```python
from build123d import *

# Parameters (mm, degrees)
F0_R     = 0.8
F0_R_2   = 1.5
F0_R_3   = 1.25
F1_DEPTH = 2


with BuildPart() as f1:
    # F0 (on Top) → F1 (new body)
    with BuildSketch(Plane.XY):
        with BuildLine():
            Line((10.009608, -5.875233), (10.009608, 5.875233))
            ThreePointArc((10.009608, 5.875233), (10.10321, 6.479919), (10.375253, 7.028005))
            Line((10.375253, 7.028005), (11.773889, 8.782295))
            ThreePointArc((11.773889, 8.782295), (12.209984, 10.04744), (11.750731, 11.304364))
            Line((11.750731, 11.304364), (10.320118, 13.032675))
            ThreePointArc((10.320118, 13.032675), (10.044588, 13.582548), (9.949174, 14.190143))
            Line((9.949174, 14.190143), (8.682091, 25.56351))
            ThreePointArc((8.682091, 25.56351), (8.678182, 25.607343), (8.676205, 25.651306))
            ThreePointArc((8.676205, 25.651306), (6.95314, 27.312167), (5.276671, 25.604284))
            ThreePointArc((5.276671, 25.604284), (5.276621, 25.588507), (5.276322, 25.572732))
            Line((5.276322, 25.572732), (5.024577, 16.189424))
            ThreePointArc((5.024577, 16.189424), (4.40399, 14.772505), (2.970938, 14.190143))
            Line((2.970938, 14.190143), (-2.970938, 14.190143))
            ThreePointArc((-2.970938, 14.190143), (-4.40399, 14.772505), (-5.024577, 16.189424))
            Line((-5.024577, 16.189424), (-5.276322, 25.572732))
            ThreePointArc((-5.276322, 25.572732), (-5.276621, 25.588507), (-5.276671, 25.604284))
            ThreePointArc((-5.276671, 25.604284), (-6.95314, 27.312167), (-8.676205, 25.651306))
            ThreePointArc((-8.676205, 25.651306), (-8.678182, 25.607343), (-8.682091, 25.56351))
            Line((-8.682091, 25.56351), (-9.949174, 14.190143))
            ThreePointArc((-9.949174, 14.190143), (-10.044588, 13.582548), (-10.320118, 13.032675))
            Line((-10.320118, 13.032675), (-11.750731, 11.304364))
            ThreePointArc((-11.750731, 11.304364), (-12.209984, 10.04744), (-11.773889, 8.782295))
            Line((-11.773889, 8.782295), (-10.375253, 7.028005))
            ThreePointArc((-10.375253, 7.028005), (-10.10321, 6.479919), (-10.009608, 5.875233))
            Line((-10.009608, 5.875233), (-10.009608, -5.875233))
            ThreePointArc((-10.009608, -5.875233), (-10.10321, -6.479919), (-10.375253, -7.028005))
            Line((-10.375253, -7.028005), (-11.773889, -8.782295))
            ThreePointArc((-11.773889, -8.782295), (-12.209984, -10.04744), (-11.750731, -11.304364))
            Line((-11.750731, -11.304364), (-10.320118, -13.032675))
            Line((-10.320118, -13.032675), (-2.368045, -22.639501))
            ThreePointArc((-2.368045, -22.639501), (-2.11021, -23.039914), (-1.954354, -23.489934))
            ThreePointArc((-1.954354, -23.489934), (0, -25.065081), (1.954354, -23.489934))
            ThreePointArc((1.954354, -23.489934), (2.11021, -23.039914), (2.368045, -22.639501))
            Line((2.368045, -22.639501), (10.320118, -13.032675))
            Line((10.320118, -13.032675), (11.750731, -11.304364))
            ThreePointArc((11.750731, -11.304364), (12.209984, -10.04744), (11.773889, -8.782295))
            Line((11.773889, -8.782295), (10.375253, -7.028005))
            ThreePointArc((10.375253, -7.028005), (10.10321, -6.479919), (10.009608, -5.875233))
        make_face()
        with Locations((0, -23.06508)):
            Circle(F0_R, mode=Mode.SUBTRACT)
        with BuildLine():
            Line((-4.566131, -18.556385), (-7.499292, -15.01286))
            ThreePointArc((-7.499292, -15.01286), (-7.544344, -14.866566), (-7.472755, -14.731265))
            Line((-7.472755, -14.731265), (-7.010556, -14.348679))
            ThreePointArc((-7.010556, -14.348679), (-6.864262, -14.303627), (-6.728961, -14.375216))
            Line((-6.728961, -14.375216), (-3.7958, -17.918741))
            ThreePointArc((-3.7958, -17.918741), (-3.750748, -18.065034), (-3.822337, -18.200336))
            Line((-3.822337, -18.200336), (-4.284536, -18.582922))
            ThreePointArc((-4.284536, -18.582922), (-4.43083, -18.627974), (-4.566131, -18.556385))
        make_face(mode=Mode.SUBTRACT)
        with Locations((0, -18.439241)):
            Circle(F0_R_2, mode=Mode.SUBTRACT)
        with Locations((-10, -10)):
            Circle(F0_R_3, mode=Mode.SUBTRACT)
        with BuildLine():
            ThreePointArc((5, -8.632429), (4.707107, -9.339536), (4, -9.632429))
            Line((4, -9.632429), (-4, -9.632429))
            ThreePointArc((-4, -9.632429), (-4.707107, -9.339536), (-5, -8.632429))
            Line((-5, -8.632429), (-5, -0.632429))
            ThreePointArc((-5, -0.632429), (-4.707107, 0.074678), (-4, 0.367571))
            Line((-4, 0.367571), (4, 0.367571))
            ThreePointArc((4, 0.367571), (4.707107, 0.074678), (5, -0.632429))
            Line((5, -0.632429), (5, -8.632429))
        make_face(mode=Mode.SUBTRACT)
        with BuildLine():
            Line((3.7958, -17.918741), (6.728961, -14.375216))
            ThreePointArc((6.728961, -14.375216), (6.864262, -14.303627), (7.010556, -14.348679))
            Line((7.010556, -14.348679), (7.472755, -14.731265))
            ThreePointArc((7.472755, -14.731265), (7.544344, -14.866566), (7.499292, -15.01286))
            Line((7.499292, -15.01286), (4.566131, -18.556385))
            ThreePointArc((4.566131, -18.556385), (4.43083, -18.627974), (4.284536, -18.582922))
            Line((4.284536, -18.582922), (3.822337, -18.200336))
            ThreePointArc((3.822337, -18.200336), (3.750748, -18.065034), (3.7958, -17.918741))
        make_face(mode=Mode.SUBTRACT)
        with Locations((10, -10)):
            Circle(F0_R_3, mode=Mode.SUBTRACT)
        with Locations((-10.009608, 10.009608)):
            Circle(F0_R_3, mode=Mode.SUBTRACT)
        with Locations((-6.976652, 25.61233)):
            Circle(F0_R, mode=Mode.SUBTRACT)
        with Locations((10.009608, 10.009608)):
            Circle(F0_R_3, mode=Mode.SUBTRACT)
        with Locations((6.976652, 25.61233)):
            Circle(F0_R, mode=Mode.SUBTRACT)
    extrude(amount=F1_DEPTH)


solid = f1.part
```
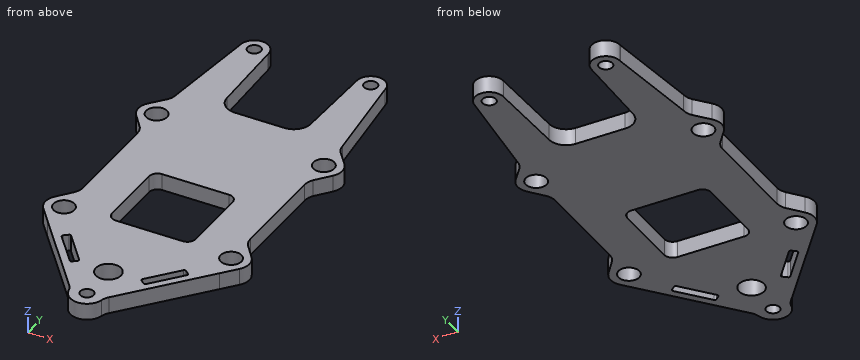
The listing builds one solid part. Answer for the finished solid, in the listing's coordinates (mm). Round coordinates to 2 decimals unless told otherwise and drop trailing zeros. Order: outer loops, then holes, each group sorted by start corner. A loop starts at its lowest first (then second) coordinate and runs counter-clockwise, first axis right, second up. Notation, with made-up numbers: (57, -15) - (78, -15) arc R13 cw to (78, -10) - close; hole circle Ø8 at (-8.5, 5.5). An arc over 180 degrees is marked (long way). Put each result on its own line as item: value. Start each with the question number.
(1) Straight lines are drawn through the part: probe 1 along Y at (x, z) = (0, 1.45); probe 2 along X at (y, z) = (25, 0.25); probe 3 along X at (y, z) = (11, 1.95). For each, find the intervals that lie inside material, in ascending order. Write a range as from..to.
(2) Find section C-C (y = -15.5). Give the vertices of the cut face in (x, z).
(3) Given P1, Ø1, axis at x = -4.5, z = 1, coming from the -Y side; P2, Ø1, axis at y = -6.5, z = 0.5, coming from the +X side; P3, Ø1.3, axis at x = 6.98, y = 25.61, coming from the -Z side; P4, Ø0.6, axis at y = 0, z = 1, coming from the +X side, each flat-ended and moving along its own axis, determine where each tip first touches the part or whether it passes through.
(4) Find section B-B (y = 15.5). Give the vertices of the cut face in (x, z).
(5) Find section A-A (x = 0). Give the vertices of the cut face in (y, z), plus the area to 3 significant figures.
(6) Find section D-D (x = -9.25). Give the vertices of the cut face in (y, z), plus the area to 3 significant figures.
Reply:
1. probe 1: -25.07..-23.87, -22.27..-19.94, -16.94..-9.63, 0.37..14.19
1. probe 2: -8.74..-7.49, -6.46..-5.26, 5.26..6.46, 7.49..8.74
1. probe 3: -11.96..-10.77, -9.25..9.25, 10.77..11.96
2. outline: (-8.28, 0) - (-7.1, 0) - (-7.1, 2) - (-8.28, 2) - close; (-5.8, 0) - (5.8, 0) - (5.8, 2) - (-5.8, 2) - close; (7.1, 0) - (8.28, 0) - (8.28, 2) - (7.1, 2) - close
3. P1: y = -20.67
3. P2: x = 10.36
3. P3: through
3. P4: x = 10.01
4. outline: (-9.8, 0) - (-4.89, 0) - (-4.89, 2) - (-9.8, 2) - close; (4.89, 0) - (9.8, 0) - (9.8, 2) - (4.89, 2) - close
5. outline: (-25.07, 0) - (-23.87, 0) - (-23.87, 2) - (-25.07, 2) - close; (-22.27, 0) - (-19.94, 0) - (-19.94, 2) - (-22.27, 2) - close; (-16.94, 0) - (-9.63, 0) - (-9.63, 2) - (-16.94, 2) - close; (0.37, 0) - (14.19, 0) - (14.19, 2) - (0.37, 2) - close
5. area: 49.3 mm^2
6. outline: (-14.33, 0) - (-11, 0) - (-11, 2) - (-14.33, 2) - close; (-9, 0) - (9.02, 0) - (9.02, 2) - (-9, 2) - close; (11, 0) - (20.47, 0) - (20.47, 2) - (11, 2) - close
6. area: 61.6 mm^2
